from build123d import *

# Parameters (mm, degrees)
F1_DEPTH       = 5
F3_D           = 3.5
F3_CSINK_D     = 7
F3_CSINK_ANGLE = 90
F4_D           = 3.5
F4_CSINK_D     = 7
F4_CSINK_ANGLE = 90
F5_R           = 5
F6_R           = 1


with BuildPart() as f1:
    # F0 (on Front) → F1 (new body, symmetric)
    with BuildSketch(Plane.XZ):
        Polygon((-4.15, 12.126713), (0, 12.126713), (4.15, 12.126713), (4.15, -30.373287), (19.15, -30.373287), (19.15, -25.373287), (9.15, -25.373287), (9.15, 17.126713), (0, 17.126713), (-9.15, 17.126713), (-9.15, -25.373287), (-19.15, -25.373287), (-19.15, -30.373287), (-4.15, -30.373287), align=None)
    extrude(amount=F1_DEPTH, both=True)

    # F3 (through all)
    with Locations(Plane.XY.offset(-25.373287)):
        with Locations((13.293465, 0)):
            CounterSinkHole(F3_D / 2, F3_CSINK_D / 2, counter_sink_angle=F3_CSINK_ANGLE)

    # F4 (through all)
    with Locations(Plane.XY.offset(-25.373287)):
        with Locations((-14.15, 0)):
            CounterSinkHole(F4_D / 2, F4_CSINK_D / 2, counter_sink_angle=F4_CSINK_ANGLE)

    # F5
    f5_edges = [f1.edges().sort_by_distance(p)[0] for p in [
        (-9.15, 0, 17.126713),
        (9.15, 0, 17.126713),
    ]]
    fillet(f5_edges, radius=F5_R)

    # F6
    f6_edges = [f1.edges().sort_by_distance(p)[0] for p in [
        (19.15, 5, -27.873287),
        (19.15, -5, -27.873287),
        (-19.15, -5, -27.873287),
        (-19.15, 5, -27.873287),
    ]]
    fillet(f6_edges, radius=F6_R)


solid = f1.part
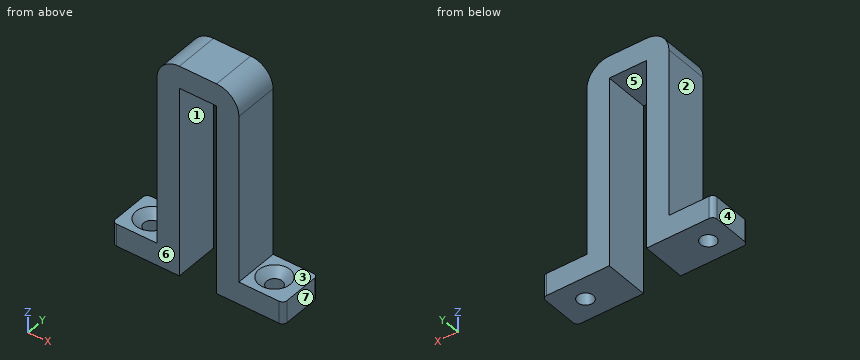
Can you work these out from the model? Positions are in its coordinate system, mm. Face numbers are marked on the shaded views. A direction names the side the tool comes from. Round coordinates to 2 decimals unless told otherwise and drop trailing zeros. Loops run counter-clockwise (first coordinate to the right, second up) from the corner with the lowest first, then second, coordinate; pieces in that order, holes last. Notation, with made-up numbers: (-30.75, -26) - (-20.75, -26) arc R31 cw to (-20.75, 8) - close; hole circle Ø9 at (34.25, 38.5). An arc over 180 degrees is marked (long way). Answer in a Markdown table with one row per item. Add a question column.
Q1. I want a section at B-B on x = -14.15. List the corners of the cut face in (y, z) for me, and give its area (3 significant figures).
Q2. We'd pull the mould along X, two halves only. Please class the marked faces 5, 6 and 7: pulls with the +X half, pulls with the -X half, needs draft (parallel to the pull), parting line crosses it, or undercut.
Q3. For pin 1 Ø5 at (y, z) = (1.5, -16) entering from +X; pin 2 Ø1 at (x, y) = (12, 1) entering from +Z; pin 3 Ø5.5 at (x, y) = (-14.15, 0) entering from -Z; pin 4 Ø1.5 at (x, z) = (-2, -5) entering from -Y, each with a flat end and sliding along its axis, tell me the tip position at first contact or that it passes through.
Q4. Which directions (+Z, -Z, +X, -X, +Y, -Y) give clear straight access to the entire face, cutting with the end or side of a thin tool? Please do the marked faces 1, 2, 3 and 4.
Q5. I want a section at D-D on z = -12. List the corners of the cut face in (x, y) for me.
Q6. I need wall thicknesses on L1, parallel to X at y = 0, z = -29.45; L2, parallel to X at y = -2.5, z = -23; L3, parallel to Y at x = -14.15, z = -28.3. Which ranges of each line are inside material? Lowest first, please.
Q7. I want a section at A-A on y = 0. List the corners of the cut face in (x, z) for me, and give its area (3 significant figures).
Q8. I want a section at C-C on z = -26. List the corners of the cut face in (x, y) for me.
A:
| question | item | result |
|---|---|---|
| 1 | outline | (-5, -30.37) - (-1.75, -30.37) - (-1.75, -27.12) - (-3.5, -25.37) - (-5, -25.37) - close; (1.75, -30.37) - (5, -30.37) - (5, -25.37) - (3.5, -25.37) - (1.75, -27.12) - close |
| 1 | area | 29.4 mm^2 |
| 2 | face 5 | undercut |
| 2 | face 6 | needs draft |
| 2 | face 7 | pulls with the +X half |
| 3 | pin 1 | x = 9.15 |
| 3 | pin 2 | z = -26.74 |
| 3 | pin 3 | z = -30.37 |
| 3 | pin 4 | through |
| 4 | face 1 | -Z, +Y, -Y |
| 4 | face 2 | +Z, -X, +Y, -Y |
| 4 | face 3 | +Z, +X, +Y, -Y |
| 4 | face 4 | +Z, -Z, -X, +Y, -Y |
| 5 | outline | (-9.15, -5) - (-4.15, -5) - (-4.15, 5) - (-9.15, 5) - close; (4.15, -5) - (9.15, -5) - (9.15, 5) - (4.15, 5) - close |
| 6 | L1 | -19.15 to -15.9, -12.4 to -4.15, 4.15 to 11.54, 15.04 to 19.15 |
| 6 | L2 | -9.15 to -4.15, 4.15 to 9.15 |
| 6 | L3 | -5 to -1.75, 1.75 to 5 |
| 7 | outline | (-19.15, -30.37) - (-15.9, -30.37) - (-15.9, -27.12) - (-17.65, -25.37) - (-19.15, -25.37) - close; (-12.4, -30.37) - (-4.15, -30.37) - (-4.15, 12.13) - (4.15, 12.13) - (4.15, -30.37) - (11.54, -30.37) - (11.54, -27.12) - (9.79, -25.37) - (9.15, -25.37) - (9.15, 12.13) arc R5 ccw to (4.15, 17.13) - (-4.15, 17.13) arc R5 ccw to (-9.15, 12.13) - (-9.15, -25.37) - (-10.65, -25.37) - (-12.4, -27.12) - close; (15.04, -30.37) - (19.15, -30.37) - (19.15, -25.37) - (16.79, -25.37) - (15.04, -27.12) - close |
| 7 | area | 565 mm^2 |
| 8 | outline | (-19.15, -4) arc R1 ccw to (-18.15, -5) - (-4.15, -5) - (-4.15, 5) - (-18.15, 5) arc R1 ccw to (-19.15, 4) - close; (4.15, -5) - (18.15, -5) arc R1 ccw to (19.15, -4) - (19.15, 4) arc R1 ccw to (18.15, 5) - (4.15, 5) - close; hole circle Ø5.75 at (-14.15, 0); hole circle Ø5.75 at (13.29, 0) |
